Geometry: final body of the model. Coordinates: model frame, mm. A direction names the side the tool comes from. Give positions to 0.01 mm unless a question says otherwise; leave off trailing zeros. Order: outer loops, then holes, each group sorted by start corner. A loop starts at its lowest first (then second) coordinate and runs counter-clockwise, first axis right, second up. Notation, with made-up numbers: (-26, 69.5) -> (9, 69.5) arc R15 ccw to (9, 75.5) -> close; hole circle Ø9 at (-34, 76). An arc over 180 degrees is marked (long way). One line per question, with ' | ' between items.
from build123d import *

# Parameters (mm, degrees)
ESBO_O1_W                = 5
ESBO_O1_H                = 4.25
ESBO_O2_R                = 2.5
RESSALTO_EXTRUS_O1_DEPTH = 16
CORTE_EXTRUS_O1_DEPTH    = 2.5
CHANFRO1_SIZE            = 0.3
FILETE1_R                = 0.2


with BuildPart() as part:
    # Esboço1 → Revolução1 (revolve)
    with BuildSketch(Plane(origin=(0, 0, 0), x_dir=(-1, 0, 0), z_dir=(0, 0, -1)), mode=Mode.PRIVATE) as revolu_o1_sk:
        with Locations((-2.5, 2.125)):
            Rectangle(ESBO_O1_W, ESBO_O1_H)
    revolve(revolu_o1_sk.sketch.rotate(Axis((5, 0, 0), (-1, 0, 0)), 270), axis=Axis((5, 0, 0), (-1, 0, 0)))

    # Esboço2 → Ressalto-extrusão1 (add)
    with BuildSketch(Plane(origin=(5, 0, 0), x_dir=(0, 0, -1), z_dir=(1, 0, 0))):
        Circle(ESBO_O2_R)
    extrude(amount=RESSALTO_EXTRUS_O1_DEPTH)

    # Esboço3 → Corte-extrusão1 (cut)
    with BuildSketch(Plane.ZY):
        Polygon((0, -2.357898499), (2.042, -1.17894925), (2.042, 1.17894925), (0, 2.357898499), (-2.042, 1.17894925), (-2.042, -1.17894925), align=None)
    extrude(amount=-CORTE_EXTRUS_O1_DEPTH, mode=Mode.SUBTRACT)

    # Esboço4 → Corte-Revolução1 (revolve, cut)
    with BuildSketch(Plane.XY, mode=Mode.PRIVATE) as corte_revolu_o1_sk:
        Polygon((2.5, 2.042), (2.5, 0), (3.67894925, 0), align=None)
    revolve(corte_revolu_o1_sk.sketch.rotate(Axis((2.5, 0, 0), (1, 0, 0)), 90), axis=Axis((2.5, 0, 0), (1, 0, 0)), mode=Mode.SUBTRACT)

    # Chanfro1
    chanfro1_edges = [part.edges().sort_by_distance(p)[0] for p in [
        (21, 0, 2.5),
        (0, 0, -4.25),
    ]]
    chamfer(chanfro1_edges, length=CHANFRO1_SIZE)

    # Filete1
    filete1_edges = [part.edges().sort_by_distance(p)[0] for p in [
        (5, 0, 2.5),
    ]]
    fillet(filete1_edges, radius=FILETE1_R)

    # Sketch1 → Cut-Revolve1 (revolve, cut)
    with BuildSketch(Plane(origin=(0, 0, 0), x_dir=(1, 0, 0), z_dir=(0, 1, 0))):
        Polygon((0, 2.36), (1.362546635, 0), (0, 0), align=None)
    revolve(axis=Axis((1.362546635, 0, 0), (1, 0, 0)), mode=Mode.SUBTRACT)


solid = part.part
1) Section A-A on x = 2.25. Return loops of the section in (y, z), plus the area to 3 significant figures.
Check result:
outline: circle Ø8.5 at (0, 0); hole (-2.36, 0) -> (-1.18, -2.04) -> (1.18, -2.04) -> (2.36, 0) -> (1.18, 2.04) -> (-1.18, 2.04) -> close | area: 42.3 mm^2
2) Contact query for flat-ended pins moving along their axis: pin 1 Ø1 at (x, z) = (16, -1.5) entering from -Y; pin 2 Ø3 at (x, y) = (18, 1.5) entering from -Z; pin 3 Ø1.5 at (x, z) = (14.5, 0) entering from -Y. Output: stop coordinate, or through.
Check result:
pin 1: stops at y = -2.29 | pin 2: stops at z = -2.5 | pin 3: stops at y = -2.5
3) Material intervals for probe 1 along X at (y, z) = (2.5, -1); probe 2 along Z at (x, y) = (1.5, 1); probe 3 along X at (y, z) = (1.25, 1.75), sorted ascending. Write a range as from..to.
Check result:
probe 1: x = 0..5 | probe 2: z = -4.13..-2.04, 2.04..4.13 | probe 3: x = 2.5..21
4) Section B-B on x = 10.75. Return loops of the section in (y, z).
Check result:
outline: circle Ø5 at (0, 0)
5) Set-up query: faces 1 (the flat face through (1.233, -1.777, 1.007)), 2 (the flat face through (5, -3, 0)), 3 (the cylindrical face through (2.617, 4.214, -0.553)). Return all of +Z, -Z, +X, -X, +Y, -Y with unobstructed straight access to the full face (end or side cutting, diameter ignored); none if empty.
Check result:
face 1: -X | face 2: +X | face 3: +X, -X
6) Pull-direction query (Z, two-part tool) for faces 4 (the flat face through (21, 0, 0)), 5 (the conical face through (3.474, 0.216, -0.281)), 6 (the cylindrical face through (12.84, -2.44, 0.54)); classes: +Z half, -Z half, draft (parallel to the pull), parting line (faces both ways), or undercut.
Check result:
face 4: draft | face 5: undercut | face 6: parting line
